from build123d import *

# Parameters (mm, degrees)
SKETCH1_W           = 100
SKETCH1_H           = 204
BOSS_EXTRUDE1_DEPTH = 3
SKETCH2_W           = 10
SKETCH2_H           = 3
BOSS_EXTRUDE2_DEPTH = 3
LPATTERN1_COUNT     = 5
LPATTERN1_PITCH     = 20
SKETCH3_W           = 10
SKETCH3_H           = 3
BOSS_EXTRUDE3_DEPTH = 3
LPATTERN2_COUNT     = 5
LPATTERN2_PITCH     = 20
SKETCH4_W           = 3
SKETCH4_H           = 10
CUT_EXTRUDE1_DEPTH  = 4
LPATTERN3_COUNT     = 10
LPATTERN3_PITCH     = 20
SKETCH5_R           = 1.1
SKETCH5_W           = 36
SKETCH5_H           = 30
CUT_EXTRUDE2_DEPTH  = 4
SKETCH6_W           = 12
SKETCH6_H           = 3
SKETCH6_W_2         = 10
BOSS_EXTRUDE4_DEPTH = 3


with BuildPart() as part:
    # Sketch1 → Boss-Extrude1 (new body)
    with BuildSketch(Plane(origin=(0, 0, 0), x_dir=(1, 0, 0), z_dir=(0, 1, 0))):
        with Locations((50, 102)):
            Rectangle(SKETCH1_W, SKETCH1_H)
    extrude(amount=BOSS_EXTRUDE1_DEPTH)

    # Sketch2 → Boss-Extrude2 (add)
    with BuildSketch(Plane.XY):
        with Locations((95, 1.5)):
            Rectangle(SKETCH2_W, SKETCH2_H)
    boss_extrude2 = extrude(amount=BOSS_EXTRUDE2_DEPTH)

    # LPattern1: Boss-Extrude2 ×5
    with Locations(*[(-i * LPATTERN1_PITCH, 0, 0) for i in range(1, LPATTERN1_COUNT)]):
        add(boss_extrude2)

    # Sketch3 → Boss-Extrude3 (add)
    with BuildSketch(Plane(origin=(0, 0, -204), x_dir=(-1, 0, 0), z_dir=(0, 0, -1))):
        with Locations((-95, 1.5)):
            Rectangle(SKETCH3_W, SKETCH3_H)
    boss_extrude3 = extrude(amount=BOSS_EXTRUDE3_DEPTH)

    # LPattern2: Boss-Extrude3 ×5
    with Locations(*[(-i * LPATTERN2_PITCH, 0, 0) for i in range(1, LPATTERN2_COUNT)]):
        add(boss_extrude3)

    # Sketch4 → Cut-Extrude1 (cut, through all)
    with BuildSketch(Plane(origin=(0, 3, 0), x_dir=(1, 0, 0), z_dir=(0, 1, 0))):
        with Locations((46.5, 12)):
            Rectangle(SKETCH4_W, SKETCH4_H)
    cut_extrude1 = extrude(amount=-CUT_EXTRUDE1_DEPTH, mode=Mode.SUBTRACT)

    # LPattern3: Cut-Extrude1 ×10
    with Locations(*[(0, 0, -i * LPATTERN3_PITCH) for i in range(1, LPATTERN3_COUNT)]):
        add(cut_extrude1, mode=Mode.SUBTRACT)

    # Sketch5 → Cut-Extrude2 (cut, through all)
    with BuildSketch(Plane(origin=(0, 3, 0), x_dir=(1, 0, 0), z_dir=(0, 1, 0))):
        with Locations((88, 147.75)):
            Circle(SKETCH5_R)
        with Locations((88, 56.25)):
            Circle(SKETCH5_R)
        with Locations((16, 56.25)):
            Circle(SKETCH5_R)
        with Locations((16, 147.75)):
            Circle(SKETCH5_R)
        with Locations((74, 20)):
            Rectangle(SKETCH5_W, SKETCH5_H)
        with Locations((74, 184)):
            Rectangle(SKETCH5_W, SKETCH5_H)
    extrude(amount=-CUT_EXTRUDE2_DEPTH, mode=Mode.SUBTRACT)

    # Sketch6 → Boss-Extrude4 (add)
    with BuildSketch(Plane(origin=(100, 0, 0), x_dir=(0, 0, -1), z_dir=(1, 0, 0))):
        with Locations((198, 1.5)):
            Rectangle(SKETCH6_W, SKETCH6_H)
        with Locations((157, 1.5)):
            Rectangle(SKETCH6_W_2, SKETCH6_H)
        with Locations((177, 1.5)):
            Rectangle(SKETCH6_W_2, SKETCH6_H)
        with Locations((137, 1.5)):
            Rectangle(SKETCH6_W_2, SKETCH6_H)
        with Locations((117, 1.5)):
            Rectangle(SKETCH6_W_2, SKETCH6_H)
        with Locations((97, 1.5)):
            Rectangle(SKETCH6_W_2, SKETCH6_H)
        with Locations((77, 1.5)):
            Rectangle(SKETCH6_W_2, SKETCH6_H)
        with Locations((57, 1.5)):
            Rectangle(SKETCH6_W_2, SKETCH6_H)
        with Locations((37, 1.5)):
            Rectangle(SKETCH6_W_2, SKETCH6_H)
        with Locations((17, 1.5)):
            Rectangle(SKETCH6_W_2, SKETCH6_H)
    extrude(amount=BOSS_EXTRUDE4_DEPTH)


solid = part.part
Check sheet for the modelled part. Datum: model origin and axes. Units: mm. Round coordinates to 2 decimals unless told otherwise and drop trailing zeros. Loops run counter-clockwise (first coordinate to the right, second up) from the corner with the lowest first, then second, coordinate; pieces in that order, holes last.
1. Scan lines: probe 1 along X at (y, z) = (2.45, -175); probe 2 along Z at (x, y) = (88, 0.8); probe 3 along X at (y, z) = (1.7, -147.75). Record each from-to range of solid material in increasing order.
2. Sectioned sample at C-C on y = 0.7. Give the number of separate pieces and of enclosed holes in the cut face, and give its area (3 significant figures).
3. Gauge pin test, flat ends, axial feed: pin 1 Ø1.5 at (x, y) = (47, 2) entering from +Z; pin 2 Ø0.9 at (x, y) = (101.5, 1) entering from +Z; pin 3 Ø0.9 at (x, y) = (46.5, 1) entering from -Z. Record the tip position at first contact, or that the pin passes through.
4. Sectioned sample at B-B on x = 78. Record the boundary of the cut face in (y, z), and give its area (3 significant figures).
5. Sectioned sample at A-A on z = -95. Record the boundary of the cut face in (x, y), and give its area (3 significant figures).
Recorded:
1. probe 1: x = 0 to 45, 48 to 56, 92 to 103
1. probe 2: z = -204 to -199, -169 to -148.85, -146.65 to -57.35, -55.15 to -35, -5 to 0
1. probe 3: x = 0 to 14.9, 17.1 to 45, 48 to 86.9, 89.1 to 100
2. separate pieces: 1
2. enclosed holes: 16
2. area: 18,500 mm2
3. pin 1: stops at z = 0
3. pin 2: stops at z = -12
3. pin 3: stops at z = -204
4. outline: (0, -207) - (3, -207) - (3, -199) - (0, -199) - close; (0, -169) - (3, -169) - (3, -35) - (0, -35) - close; (0, -5) - (3, -5) - (3, 3) - (0, 3) - close
4. area: 450 mm2
5. outline: (0, 0) - (45, 0) - (45, 3) - (0, 3) - close; (48, 0) - (103, 0) - (103, 3) - (48, 3) - close
5. area: 300 mm2
